```python
from build123d import *

# Parameters (mm, degrees)
SKETCH1_R                  = 5
BOSS_EXTRUDE1_DEPTH        = 60
SKETCH2_W                  = 5
SKETCH2_H                  = 3
CUT_EXTRUDE1_DEPTH         = 6
BOSS_EXTRUDE2_REACH        = 65.415
BOSS_EXTRUDE2_START_RADIUS = 5
BOSS_EXTRUDE2_END_RADIUS   = 5
SKETCH4_W                  = 3
SKETCH4_H                  = 3
BOSS_EXTRUDE3_DEPTH        = 5


with BuildPart() as part:
    # Sketch1 → Boss-Extrude1 (new body)
    with BuildSketch(Plane(origin=(0, 0, 0), x_dir=(1, 0, 0), z_dir=(0, 1, 0))):
        with Locations(Location((0, 0, 0), (0, 0, 90))):
            Circle(SKETCH1_R)
    extrude(amount=BOSS_EXTRUDE1_DEPTH)

    # Sketch2 → Cut-Extrude1 (cut)
    with BuildSketch(Plane.XZ):
        Rectangle(SKETCH2_W, SKETCH2_H)
    extrude(amount=-CUT_EXTRUDE1_DEPTH, mode=Mode.SUBTRACT)

    # Boss-Extrude2: from a cylinder face, 65.415 long prism both ways, kept between that surface and its translate by the depth
    boss_extrude2_start = Plane(origin=(0, 32.976643, 0), z_dir=(0, -1, 0)) * Cylinder(BOSS_EXTRUDE2_START_RADIUS, 141.83, mode=Mode.PRIVATE)
    boss_extrude2_end = Plane(origin=(0, 32.976643, 3), z_dir=(0, -1, 0)) * Cylinder(BOSS_EXTRUDE2_END_RADIUS, 141.83, mode=Mode.PRIVATE)
    # Sketch3 → Boss-Extrude2 (add, from a surface)
    with BuildSketch(Plane.XY, mode=Mode.PRIVATE) as boss_extrude2_sk1:
        Polygon((0, 42.798210841), (-2.5, 28.065858852), (2.5, 28.065858852), align=None)
    boss_extrude2_tool1 = extrude(boss_extrude2_sk1.sketch, amount=BOSS_EXTRUDE2_REACH, both=True, mode=Mode.PRIVATE)
    add(((boss_extrude2_tool1 - boss_extrude2_start) & boss_extrude2_end).solids().sort_by_distance((0, 32.976643, 6.165064))[0])

    # Sketch4 → Boss-Extrude3 (add)
    with BuildSketch(Plane(origin=(0, 60, 0), x_dir=(1, 0, 0), z_dir=(0, 1, 0))):
        Rectangle(SKETCH4_W, SKETCH4_H)
    extrude(amount=BOSS_EXTRUDE3_DEPTH)


solid = part.part
```
The listing builds one solid part. Answer for the finished solid, in the listing's coordinates (mm). A direction names the side the tool comes from. Coordinates: 2 decimals unless noted, no trailing zeros. Loops run counter-clockwise (first coordinate to the right, second up) from the corner with the lowest first, then second, coordinate; pieces in that order, holes last. Notation, with made-up numbers: M 76,15 L 130,15 A19 cw 130,52 Z; hole C 47,8.25 d3. An arc over 180 degrees is marked long. Answer as CSV lines item,"result". Start each with the question number.
(1) The mould has two halves that part along Z. Classify faces 1 (the cylindrical face through (-1.5, 29.58, -4.77)), 2 (the flat face through (1.5, 62, 0)), 3 (the flat face through (0, 3, -1.5)), 4 (the cylindrical face through (0, 34, 8)): pulls with the +Z half, pulls with the -Z half, needs draft (parallel to the pull), parting line crosses it, or undercut.
(2) The part is cut by section A-A (z = 0). Give the vertices of the cut face in (x, y).
(3) The part is cut by section C-C (z = -3.5). Give the vertices of the cut face in (x, y).
(4) Find the intervals of material crossed by L1, parallel to Z at x = 0.25, y = 61.5; L2, parallel to Y at x = -3, z = 1.75; L3, parallel to Z at x = -0.5, y = 5, in increasing order. Write a range as [from, to].
(5) For faces 5 (the flat face through (-1.23, 35.54, 6.19)), 6 (the flat face through (-1.5, 62, 0)), 7 (the flat face through (1.267, 35.329, 6.191)), 8 (the flat face through (0, 3, 1.5)), determine the directions among +Z, -Z, +X, -X, +Y, -Y from which every point of the face is accessible in a straight line to the end or side of a thin tool.
(6) Given pin 1 (1 mm diameter, centred on y = 8, z = 4.5, fed in from +X); pin 2 (1.5 mm diameter, centred on x = 0, y = 61.5, fed in from +Z); pin 3 (2 mm diameter, centred on x = 1, y = 51.5, fed in from +Z), each flat-ended and moving along its own axis, determine where each tip first touches the part or whether it passes through.
(7) The part is cut by section B-B (y = 27.5). Give the vertices of the cut face in (x, z).
Determined:
1,face 1,"parting line crosses it"
1,face 2,"needs draft"
1,face 3,"undercut"
1,face 4,"pulls with the +Z half"
2,outline,"M -5,0 L -2.5,0 L -2.5,6 L 2.5,6 L 2.5,0 L 5,0 L 5,60 L 1.5,60 L 1.5,65 L -1.5,65 L -1.5,60 L -5,60 Z"
3,outline,"M -3.57,0 L 3.57,0 L 3.57,60 L -3.57,60 Z"
4,L1,"[-1.5, 1.5]"
4,L2,"[0, 60]"
4,L3,"[-4.97, -1.5], [1.5, 4.97]"
5,face 5,"+Z, -X, +Y"
5,face 6,"+Z, -Z, -X, +Y"
5,face 7,"+Z, +X, +Y"
5,face 8,"-Y"
6,pin 1,"x = 3"
6,pin 2,"z = 1.5"
6,pin 3,"z = 5"
7,outline,"C 0,0 d10"
